Input: dimensioned drawing with shaded views. Units: mm. Origin: part minimum x, y, z. Coordinates: 2 decimals unless noted, no trailing zeros. Loops run counter-clockwise (first coordinate to the right, second up) from the corner with the lowest first, then second, coordinate; pieces in that order, holes last.
Item 1: Contact query for a flat-ended pin moving along its axis: P1, Ø7, axis at x = 7.51, y = 6.5, coming from the -Z side. Output: stop coordinate, or through.
Item 2: Section A-A on z = 4.5. Return loops of the section in (x, y) (1 decimal).
Item 3: Pull-direction query (Y, two-part tool) for the marked faces 1, 2, 3 and 4; classes: released by +Y, released by -Y, zero draft, split by the parting line, or undercut.
Item 4: Ray query, line 1 along Y through (x, z) = (7.5, 2.75); line 2 along Y through (x, z) = (5.5, 5.5); line 3 along X through (y, z) = (3, 0.5) (1 decimal). Return the intervals inside material, ascending.
Item 5: Section B-B on z = 5.5. Return loops of the section in (x, y) (1 decimal).
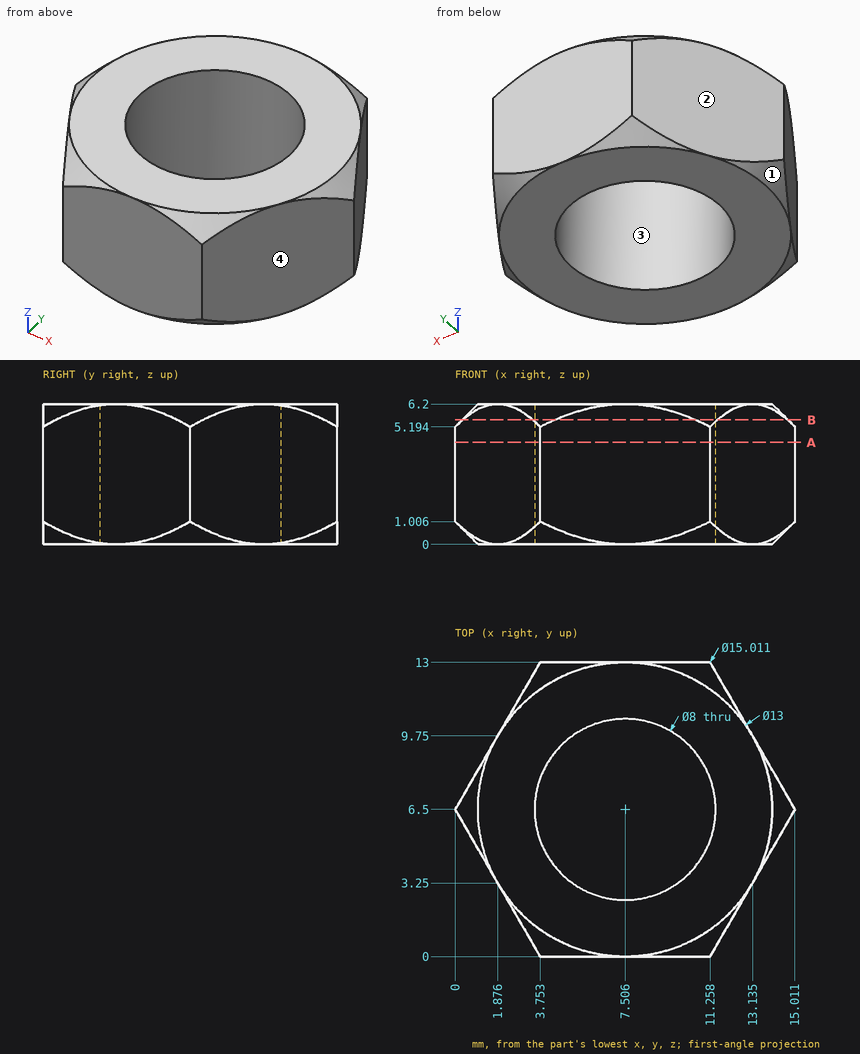
Results found:
1. P1: passes through
2. outline: (0, 6.5) - (3.8, 0) - (11.3, 0) - (15, 6.5) - (11.3, 13) - (3.8, 13) - close; hole circle Ø8 at (7.5, 6.5)
3. face 1: split by the parting line
3. face 2: released by +Y
3. face 3: undercut
3. face 4: released by -Y
4. line 1: y = 0 to 2.5, 10.5 to 13
4. line 2: y = 0 to 3.04, 9.96 to 13
4. line 3: x = 2 to 5.6, 9.4 to 13
5. outline: (0.3, 5.9) - (3.4, 0.6) arc R7.2 ccw to (4.4, 0) - (10.6, 0) arc R7.2 ccw to (11.6, 0.6) - (14.7, 5.9) arc R7.2 ccw to (14.7, 7.1) - (11.6, 12.4) arc R7.2 ccw to (10.6, 13) - (4.4, 13) arc R7.2 ccw to (3.4, 12.4) - (0.3, 7.1) arc R7.2 ccw to start; hole circle Ø8 at (7.5, 6.5)
